Design review of the part built by this model. Coordinates are the model's own, in mm. Face numbers are marked on the shaded views. A direction names the side the tool comes from. Round coordinates to 2 decimals unless told otherwise and drop trailing zeros. Order: outer loops, then holes, each group sorted by start corner. A loop starts at its lowest first (then second) coordinate and runs counter-clockwise, first axis right, second up. Notation, with made-up numbers: M 13.25,-18.5 L 68.25,-18.5 A21 cw 68.25,-2.5 Z; hole C 62,-24.5 d4. An arc over 180 degrees is marked long. Write each question's results on one line, items separated by ' | '. Start each with the question number.
Item 1: Clearance check with a flat-ended pin moving along its axis: pin 1 (1 mm diameter, centred on x = -8, y = 31, fed in from -Z). State where the tip first meets the part, or that it passes through.
Item 2: Take a section at A-A, the plane x = 0. Write out the cut boundary in (y, z).
Item 3: Take a section at C-C, the plane y = 22.5. Write out the cut boundary in (x, z) (3 decimals).
Item 4: Machinability: for the marked faces 5 and 6, which of the approach directions +Z, -Z, +X, -X, +Y, -Y give a long, thin tool a straight path to every point of the face, cutting with its end or side? Answer none if there is none.
Item 5: Take a section at D-D, the plane z = 6.25. Write out the cut boundary in (x, y) (3 decimals).
Item 6: Wall thickness on line 1 (Y direction, x = 13.5, z = 7); line 2 (Y direction, x = 0, z = 6.25); line 3 (X direction, y = 11, z = 11) (3 decimals): over which ranges is each line inside the solid? List them lowest first. Write a range as [from, to].
Item 7: The part is to be moulded in two halves that separate along Y. For the marked faces 1, 2, 3 and 4, say which applies: +Y half, -Y half, draft (parallel to the pull), parting line (faces both ways), or undercut.
Item 8: Take a section at B-B, the plane x = 14.5. Write out the cut boundary in (y, z), plus the area to 3 significant figures.
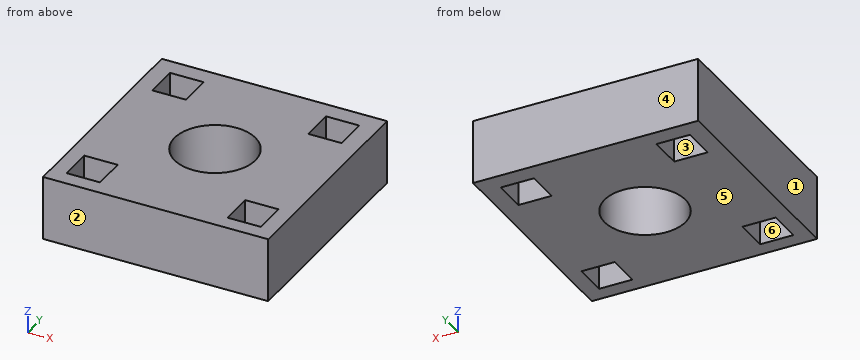
```python
from build123d import *

# Parameters (mm, degrees)
F1_DEPTH = 12.7
F2_R     = 8.001
F2_W     = 6.604
F2_H     = 6.604
F3_DEPTH = 12.7


with BuildPart() as f1:
    # F0 (on Top) → F1 (new body)
    with BuildSketch(Plane.XY):
        Polygon((22.225, 37.822188), (-22.225, 37.822188), (-22.225, -6.627812), (-5.278436, -6.627812), (12.779376, -6.627812), (22.225, -6.627812), align=None)
    extrude(amount=F1_DEPTH)

    # F2 (on face) → F3 (cut)
    with BuildSketch(Plane.XY.offset(12.7)):
        with Locations((0, 15.597188)):
            Circle(F2_R)
        with Locations((-15.459939, 31.057127)):
            Rectangle(F2_W, F2_H)
        with Locations((15.355254, 30.952442)):
            Rectangle(F2_W, F2_H)
        with Locations((15.875, -0.277812)):
            Rectangle(F2_W, F2_H)
        with Locations((-15.875, -0.277812)):
            Rectangle(F2_W, F2_H)
    extrude(amount=-F3_DEPTH, mode=Mode.SUBTRACT)


solid = f1.part
```
Results list:
1) pin 1: z = 0
2) outline: M -6.63,0 L 7.6,0 L 7.6,12.7 L -6.63,12.7 Z; M 23.6,0 L 37.82,0 L 37.82,12.7 L 23.6,12.7 Z
3) outline: M -22.225,0 L -4.046,0 L -4.046,12.7 L -22.225,12.7 Z; M 4.046,0 L 22.225,0 L 22.225,12.7 L 4.046,12.7 Z
4) face 5: -Z, +X, -X, +Y, -Y | face 6: +Z, -Z
5) outline: M -22.225,-6.628 L 22.225,-6.628 L 22.225,37.822 L -22.225,37.822 Z; hole M -19.177,-3.58 L -12.573,-3.58 L -12.573,3.024 L -19.177,3.024 Z; hole M -18.762,27.755 L -12.158,27.755 L -12.158,34.359 L -18.762,34.359 Z; hole C 0,15.597 d16.002; hole M 12.053,27.65 L 18.657,27.65 L 18.657,34.254 L 12.053,34.254 Z; hole M 12.573,-3.58 L 19.177,-3.58 L 19.177,3.024 L 12.573,3.024 Z
6) line 1: [-6.63, -3.58], [3.02, 27.65], [34.25, 37.82] | line 2: [-6.63, 7.6], [23.6, 37.82] | line 3: [-22.225, -6.548], [6.548, 22.225]
7) face 1: draft | face 2: -Y half | face 3: undercut | face 4: +Y half
8) outline: M -6.63,0 L -3.58,0 L -3.58,12.7 L -6.63,12.7 Z; M 3.02,0 L 27.65,0 L 27.65,12.7 L 3.02,12.7 Z; M 34.25,0 L 37.82,0 L 37.82,12.7 L 34.25,12.7 Z | area: 397 mm²
